from build123d import *

# Parameters (mm, degrees)
SKETCH1_R           = 16
BOSS_EXTRUDE1_DEPTH = 2
SKETCH5_R           = 2.25
CUT_EXTRUDE1_DEPTH  = 3
SKETCH6_R           = 3.975
BOSS_EXTRUDE2_DEPTH = 3
FILLET1_R           = 0.5


with BuildPart() as part:
    # Sketch1 → Boss-Extrude1 (new body)
    with BuildSketch(Plane(origin=(0, 0, 0), x_dir=(1, 0, 0), z_dir=(0, 1, 0))):
        Circle(SKETCH1_R)
    extrude(amount=BOSS_EXTRUDE1_DEPTH)

    # Sketch5 → Cut-Extrude1 (cut, through all)
    with BuildSketch(Plane(origin=(0, 2, 0), x_dir=(1, 0, 0), z_dir=(0, 1, 0))):
        with Locations((0, 12)):
            Circle(SKETCH5_R)
        with Locations((12, 0)):
            Circle(SKETCH5_R)
        with Locations((0, -12)):
            Circle(SKETCH5_R)
        with Locations((-12, 0)):
            Circle(SKETCH5_R)
    extrude(amount=-CUT_EXTRUDE1_DEPTH, mode=Mode.SUBTRACT)

    # Sketch6 → Boss-Extrude2 (add)
    with BuildSketch(Plane(origin=(0, 2, 0), x_dir=(1, 0, 0), z_dir=(0, 1, 0))):
        Circle(SKETCH6_R)
    extrude(amount=BOSS_EXTRUDE2_DEPTH)

    # Fillet1
    fillet1_edges = [part.edges().sort_by_distance(p)[0] for p in [
        (-3.975, 2, 0),
        (-3.975, 5, 0),
        (-16, 2, 0),
    ]]
    fillet(fillet1_edges, radius=FILLET1_R)


solid = part.part
Input: part model. Units: mm. Frame: model coordinates. A direction names the side the tool comes from. Round coordinates to 2 decimals unless told otherwise and drop trailing zeros. Write each loop counter-clockwise with the first axis right and the second up, starting at its lowest first coordinate (ties: lowest second). Pieces come first, ordered by that corner, then holes.
1) Contact query for flat-ended pins moving along their axis: P1, Ø4, axis at x = -12, z = 0, coming from the -Y side; P2, Ø3, axis at x = -0.5, y = 3, coming from the +Z side; P3, Ø2, axis at x = -2, z = 12, coming from the +Y side. Output: stop coordinate, or through.
2) Ray query, L1, parallel to X at y = 0.55, z = 0; L2, parallel to Z at x = 1, y = 1.55. Return the intervals inside material, ascending.
3) Cut plane A-A (x = 0). Return the cut outline in (y, z) (3 decimals).
4) Reachability of faces 4 (the cylindrical face through (-0.86, 3.49, 3.88)), 5 (the flat face through (0, 0, 0)) from +Z, -Z, +X, -X, +Y, -Y: full face, straight path, thin tool, end or side. Return the list, or none.
5) Cut plane C-C (y = 3.8). Return the cut outline in (x, z) (3 decimals), then the cut area to 3 significant figures.
6) Cut plane B-B (z = 0). Return the cut outline in (x, y) (3 decimals), then the cut area to 3 significant figures.
7) Draft query along X for faces 1 (the cylindrical face through (-3.47, 0.74, 15.62)), 2 (the flat face through (3, 2, -4)), 3 (the cylindrical face through (-0.29, 1.01, -14.23)). Return one class per face: pulls with the +X half, pulls with the -X half, needs draft (parallel to the pull), parting line crosses it, or undercut.
Geometry says:
1. P1: passes through
1. P2: stops at z = 16
1. P3: stops at y = 2
2. L1: x = -16 to -14.25, -9.75 to 9.75, 14.25 to 16
2. L2: z = -15.97 to -14.02, -9.98 to 9.98, 14.02 to 15.97
3. outline: (0, -16) - (1.5, -16) arc R0.5 ccw to (2, -15.5) - (2, -14.25) - (0, -14.25) - close; (0, -9.75) - (2, -9.75) - (2, -4.475) arc R0.5 cw to (2.5, -3.975) - (4.5, -3.975) arc R0.5 ccw to (5, -3.475) - (5, 3.475) arc R0.5 ccw to (4.5, 3.975) - (2.5, 3.975) arc R0.5 cw to (2, 4.475) - (2, 9.75) - (0, 9.75) - close; (0, 14.25) - (2, 14.25) - (2, 15.5) arc R0.5 ccw to (1.5, 16) - (0, 16) - close
4. face 4: +Y
4. face 5: +Z, -Z, +X, -X, -Y
5. outline: circle Ø7.95 at (0, 0)
5. area: 49.6 mm2
6. outline: (-16, 0) - (-14.25, 0) - (-14.25, 2) - (-15.5, 2) arc R0.5 ccw to (-16, 1.5) - close; (-9.75, 0) - (9.75, 0) - (9.75, 2) - (4.475, 2) arc R0.5 cw to (3.975, 2.5) - (3.975, 4.5) arc R0.5 ccw to (3.475, 5) - (-3.475, 5) arc R0.5 ccw to (-3.975, 4.5) - (-3.975, 2.5) arc R0.5 cw to (-4.475, 2) - (-9.75, 2) - close; (14.25, 0) - (16, 0) - (16, 1.5) arc R0.5 ccw to (15.5, 2) - (14.25, 2) - close
6. area: 69.7 mm2
7. face 1: parting line crosses it
7. face 2: needs draft
7. face 3: undercut
